from build123d import *

# Parameters (mm, degrees)
CROQUIS1_W              = 65.5
CROQUIS1_H              = 76.5
SALIENTE_EXTRUIR1_DEPTH = 1.8
CROQUIS2_W              = 5
CROQUIS2_H              = 76.5
SALIENTE_EXTRUIR2_DEPTH = 15
CORTAR_EXTRUIR1_DEPTH   = 76.5
SALIENTE_EXTRUIR4_DEPTH = 1.8
CROQUIS7_W              = 13.85
CROQUIS7_H              = 23
SALIENTE_EXTRUIR5_DEPTH = 3
CORTAR_EXTRUIR5_DEPTH   = 23
CROQUIS10_R             = 1
CORTAR_EXTRUIR6_DEPTH   = 8
CORTAR_EXTRUIR7_START   = -8
CROQUIS11_R             = 1
CORTAR_EXTRUIR7_DEPTH   = 8
CROQUIS12_R             = 1
CORTAR_EXTRUIR8_DEPTH   = 8


with BuildPart() as part:
    # Croquis1 → Saliente-Extruir1 (new body)
    with BuildSketch(Plane.XY):
        with Locations((-58.211538462, -3.442307692)):
            Rectangle(CROQUIS1_W, CROQUIS1_H)
    extrude(amount=SALIENTE_EXTRUIR1_DEPTH)

    # Croquis2 → Saliente-Extruir2 (add)
    with BuildSketch(Plane.XY.offset(1.8)):
        with Locations((-88.461538462, -3.442307692)):
            Rectangle(CROQUIS2_W, CROQUIS2_H)
        with Locations((-27.961538462, -3.442307692)):
            Rectangle(CROQUIS2_W, CROQUIS2_H)
    extrude(amount=SALIENTE_EXTRUIR2_DEPTH)

    # Croquis3 → Cortar-Extruir1 (cut)
    with BuildSketch(Plane.XZ.offset(41.692307692)):
        Polygon((-89.111538462, 15.9), (-87.811538462, 15.9), (-87.811538462, 15), (-88.461538462, 15), (-88.861538462, 15), (-88.861538462, 12.9), (-85.961538462, 12.9), (-85.961538462, 15), (-85.961538462, 16.8), (-89.111538462, 16.8), (-90.961538462, 16.8), (-90.961538462, 15.9), align=None)
        Polygon((-30.461538462, 15), (-30.461538462, 12.9), (-27.561538462, 12.9), (-27.561538462, 15), (-28.611538462, 15), (-28.611538462, 15.9), (-28.611538462, 16.8), (-30.461538462, 16.8), align=None)
    extrude(amount=-CORTAR_EXTRUIR1_DEPTH, mode=Mode.SUBTRACT)

    # Croquis6 → Saliente-Extruir4 (add)
    with BuildSketch(Plane.XZ.offset(41.692307692)):
        Polygon((-85.961538462, 7.7), (-78.961538462, 7.7), (-78.961538462, 3.5), (-45.461538462, 3.5), (-45.461538462, 7.7), (-30.461538462, 7.7), (-25.461538462, 7.7), (-25.461538462, 0), (-90.961538462, 0), (-90.961538462, 7.7), align=None)
    extrude(amount=SALIENTE_EXTRUIR4_DEPTH)

    # Croquis7 → Saliente-Extruir5 (add)
    with BuildSketch(Plane(origin=(0, 0, 0), x_dir=(-1, 0, 0), z_dir=(0, 0, -1))):
        with Locations((58.211538462, -4.342307692)):
            Rectangle(CROQUIS7_W, CROQUIS7_H)
    extrude(amount=SALIENTE_EXTRUIR5_DEPTH)

    # Croquis9 → Cortar-Extruir5 (cut)
    with BuildSketch(Plane.XZ.offset(15.842307692)):
        Polygon((-51.286538462, -3), (-54.286538462, 0), (-51.286538462, 0), align=None)
        Polygon((-65.136538462, -3), (-62.136538462, 0), (-65.136538462, 0), align=None)
    extrude(amount=-CORTAR_EXTRUIR5_DEPTH, mode=Mode.SUBTRACT)

    # Croquis10 → Cortar-Extruir6 (cut)
    with BuildSketch(Plane.XZ.offset(41.692307692)):
        with Locations(Location((-87.661538462, 10.9, 0), (0, 0, 270))):
            Circle(CROQUIS10_R)
        with Locations(Location((-29.011538462, 10.9, 0), (0, 0, 270))):
            Circle(CROQUIS10_R)
    extrude(amount=-CORTAR_EXTRUIR6_DEPTH, mode=Mode.SUBTRACT)

    # Croquis11 → Cortar-Extruir7 (cut)
    with BuildSketch(Plane(origin=(0, 34.807692308, 0), x_dir=(1, 0, 0), z_dir=(0, 1, 0)).offset(CORTAR_EXTRUIR7_START)):
        with Locations(Location((-29.011538462, -10.9, 0), (0, 0, 90))):
            Circle(CROQUIS11_R)
        with Locations(Location((-87.661538462, -10.9, 0), (0, 0, 90))):
            Circle(CROQUIS11_R)
    extrude(amount=CORTAR_EXTRUIR7_DEPTH, mode=Mode.SUBTRACT)

    # Croquis12 → Cortar-Extruir8 (cut)
    with BuildSketch(Plane(origin=(0, 34.807692308, 0), x_dir=(1, 0, 0), z_dir=(0, 1, 0))):
        with Locations(Location((-27.961538462, -2.5, 0), (0, 0, 270))):
            Circle(CROQUIS12_R)
        with Locations(Location((-88.461538462, -2.5, 0), (0, 0, 270))):
            Circle(CROQUIS12_R)
    extrude(amount=-CORTAR_EXTRUIR8_DEPTH, mode=Mode.SUBTRACT)


solid = part.part
Geometry: final body of the model. Coordinates: model frame, mm. A direction names the side the tool comes from. Round coordinates to 2 decimals unless told otherwise and drop trailing zeros. Loops run counter-clockwise (first coordinate to the right, second up) from the corner with the lowest first, then second, coordinate; pieces in that order, holes last.
Q1. Section C-C on y = 2. Return loops of the section in (x, z).
Q2. Section D-D on y = -17.5. Return loops of the section in (x, z), plus the area to 3 significant figures.
Q3. Section A-A on z = 10.9. Return loops of the section in (x, y), plus the area to 3 significant figures.
Q4. Material intervals for L1, parallel to X at y = -38.25, z = 10.9; L2, parallel to X at y = 32.5, z = 2.5; L3, parallel to X at y = -20, z = 12.75, sorted ascending.
Q5. Pin query (flat end, axial travel): P1, Ø1, axis at x = -87.5, z = 10.5, coming from the -Y side; P2, Ø1.4, axis at x = -85, y = -42.5, coming from the +Z side; P3, Ø4, axis at x = -47, y = -18.5, coming from the -Z side; P4, Ø5, axis at x = -65.5, z = 8, coming from the -Y side. Return the tip coordinate at first contact, or that it passes through.
Q6. Section B-B on x = -56. Return loops of the section in (y, z).
Q7. Access query for faces 3 (the flat face through (-27.562, -4, 14)), 4 (the cylindrical face through (-29.855, 30.752, 10.362)), 5 (the flat face through (-89, -41.692, 11)). Directions: +Z, -Z, +X, -X, +Y, -Y. A direction counts if a zero-diameter tool reaches every point of the face in a straight line with its end or side. Return the directions, or none.
Q8. Pull-direction query (X, two-part tool) for faces 1 (the cylindrical face through (-29.9, -37.75, 10.44)), 2 (the flat face through (-58, -15.842, -1)); classes: released by +X, released by -X, zero draft, split by the parting line, or undercut.
Evaluation:
1. outline: (-90.96, 0) - (-62.14, 0) - (-65.14, -3) - (-51.29, -3) - (-54.29, 0) - (-25.46, 0) - (-25.46, 16.8) - (-28.61, 16.8) - (-28.61, 15) - (-27.56, 15) - (-27.56, 12.9) - (-30.46, 12.9) - (-30.46, 1.8) - (-85.96, 1.8) - (-85.96, 12.9) - (-88.86, 12.9) - (-88.86, 15) - (-87.81, 15) - (-87.81, 15.9) - (-90.96, 15.9) - close
2. outline: (-90.96, 0) - (-25.46, 0) - (-25.46, 16.8) - (-28.61, 16.8) - (-28.61, 15) - (-27.56, 15) - (-27.56, 12.9) - (-30.46, 12.9) - (-30.46, 1.8) - (-85.96, 1.8) - (-85.96, 12.9) - (-88.86, 12.9) - (-88.86, 15) - (-87.81, 15) - (-87.81, 15.9) - (-90.96, 15.9) - close
2. area: 246 mm2
3. outline: (-90.96, -41.69) - (-88.66, -41.69) - (-88.66, -33.69) - (-86.66, -33.69) - (-86.66, -41.69) - (-85.96, -41.69) - (-85.96, 34.81) - (-86.66, 34.81) - (-86.66, 26.81) - (-88.66, 26.81) - (-88.66, 34.81) - (-90.96, 34.81) - close; (-30.46, -41.69) - (-30.01, -41.69) - (-30.01, -33.69) - (-28.01, -33.69) - (-28.01, -41.69) - (-25.46, -41.69) - (-25.46, 34.81) - (-28.01, 34.81) - (-28.01, 26.81) - (-30.01, 26.81) - (-30.01, 34.81) - (-30.46, 34.81) - close
3. area: 701 mm2
4. L1: x = -90.96 to -88.66, -86.66 to -85.96, -30.46 to -30.01, -28.01 to -25.46
4. L2: x = -90.96 to -89.46, -87.46 to -85.96, -30.46 to -28.96, -26.96 to -25.46
4. L3: x = -90.96 to -85.96, -30.46 to -25.46
5. P1: stops at y = -33.69
5. P2: stops at z = 7.7
5. P3: stops at z = 0
5. P4: passes through
6. outline: (-43.49, 0) - (-15.84, 0) - (-15.84, -3) - (7.16, -3) - (7.16, 0) - (34.81, 0) - (34.81, 1.8) - (-41.69, 1.8) - (-41.69, 3.5) - (-43.49, 3.5) - close
7. face 3: +Y, -Y
7. face 4: +Y
7. face 5: +Z, +X, -X, -Y
8. face 1: undercut
8. face 2: zero draft
